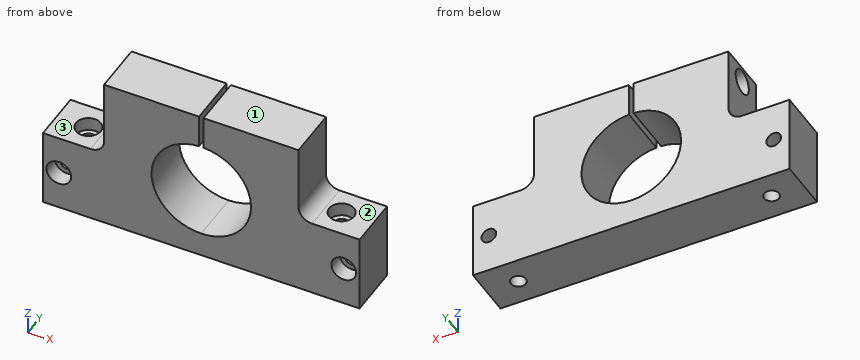
from build123d import *

# Parameters (mm, degrees)
DODANIE_WYCI_GNI_CIE1_DEPTH                        = 23
ZAOKR_GLENIE1_R                                    = 6
POG_BIENIE_START                                   = 27
POG_BIENIE_WALCOWE_POD_M6_WKR_T_DO_C_2_R           = 3.25
POG_BIENIE_WALCOWE_POD_M6_WKR_T_DO_CZ_CI_DEPTH     = 42
POG_BIENIE_WALCOWE_POD_M6_WKR_T_DO_C_3_O_R         = 5.5
POG_BIENIE_WALCOWE_POD_M6_WKR_T_DO_C_3_O_R_2       = 3.25
POG_BIENIE_WALCOWE_POD_M6_WKR_T_DO_C_3_DEPTH       = 7
OTW_R_GWINTOWANY_M6X1_01_D                         = 5
OTW_R_GWINTOWANY_M6X1_01_DEPTH                     = 17
OTW_R_GWINTOWANY_M6X1_01_TIP                       = 1.502151548
POG_BIENIE_WALCOWE_POD_M6_WKR_T_DO_C_4_D           = 6.6
POG_BIENIE_WALCOWE_POD_M6_WKR_T_DO_C_4_CBORE_D     = 11
POG_BIENIE_WALCOWE_POD_M6_WKR_T_DO_C_4_CBORE_DEPTH = 6
POG_BIENIE_WALCOWE_POD_M6_WKR_T_DO_C_5_D           = 6.5
POG_BIENIE_WALCOWE_POD_M6_WKR_T_DO_C_5_CBORE_D     = 11
POG_BIENIE_WALCOWE_POD_M6_WKR_T_DO_C_5_CBORE_DEPTH = 7


# Read off the part's stored shape, not the designer's step: Pogłębienie walcowe pod M6 Wkręt do części metalowych z łbem sześciokątnym1
with BuildPart() as part:
    # Szkic1 → Dodanie-wyciągnięcie1 (new body)
    with BuildSketch(Plane(origin=(0, 0, 0), x_dir=(1, 0, 0), z_dir=(0, 1, 0))):
        with BuildLine():
            Line((0, 0), (0, -35))
            Line((0, -35), (27, -35))
            Line((27, -35), (27, -70))
            Line((27, -70), (69, -70))
            Line((69, -70), (69, -54.977260976))
            ThreePointArc((69, -54.977260976), (48.005685491, -32.499870751), (70, -11))
            Line((70, -11), (70, 0))
            Line((70, 0), (0, 0))
        make_face()
        with BuildLine():
            Line((140, 0), (70, 0))
            Line((70, 0), (70, -11))
            ThreePointArc((70, -11), (91.994314509, -32.499870751), (71, -54.977260976))
            Line((71, -54.977260976), (71, -70))
            Line((71, -70), (113, -70))
            Line((113, -70), (113, -35))
            Line((113, -35), (140, -35))
            Line((140, -35), (140, 0))
        make_face()
    extrude(amount=DODANIE_WYCI_GNI_CIE1_DEPTH)

    # Zaokrąglenie1
    zaokr_glenie1_edges = [part.edges().sort_by_distance(p)[0] for p in [
        (27, 11.5, 35),
        (113, 11.5, 35),
    ]]
    fillet(zaokr_glenie1_edges, radius=ZAOKR_GLENIE1_R)

    # Pog_bienie walcowe pod M6 Wkr_t do c 2 → Pog_bienie walcowe pod M6 Wkr_t do cz_ci (cut)
    with BuildSketch(Plane.YZ.offset(POG_BIENIE_START)):
        with Locations((11.5, 63)):
            Circle(POG_BIENIE_WALCOWE_POD_M6_WKR_T_DO_C_2_R)
    extrude(amount=POG_BIENIE_WALCOWE_POD_M6_WKR_T_DO_CZ_CI_DEPTH, mode=Mode.SUBTRACT)

    # Pog_bienie walcowe pod M6 Wkr_t do c 3 o → Pog_bienie walcowe pod M6 Wkr_t do c 3 (cut)
    with BuildSketch(Plane.YZ.offset(POG_BIENIE_START)):
        with Locations((11.5, 63)):
            Circle(POG_BIENIE_WALCOWE_POD_M6_WKR_T_DO_C_3_O_R)
        with Locations((11.5, 63)):
            Circle(POG_BIENIE_WALCOWE_POD_M6_WKR_T_DO_C_3_O_R_2, mode=Mode.SUBTRACT)
    extrude(amount=POG_BIENIE_WALCOWE_POD_M6_WKR_T_DO_C_3_DEPTH, mode=Mode.SUBTRACT)

    # Otwór gwintowany M6x1.01
    with Locations(Plane.ZY.offset(-71)):
        with Locations((63, 11.5)):
            Hole(OTW_R_GWINTOWANY_M6X1_01_D / 2, depth=OTW_R_GWINTOWANY_M6X1_01_DEPTH)
            with Locations((0, 0, -(OTW_R_GWINTOWANY_M6X1_01_DEPTH + OTW_R_GWINTOWANY_M6X1_01_TIP / 2))):  # 118° drill point
                Cone(0, OTW_R_GWINTOWANY_M6X1_01_D / 2, OTW_R_GWINTOWANY_M6X1_01_TIP, mode=Mode.SUBTRACT)

    # Pog_bienie walcowe pod M6 Wkr_t do c 4 (through all)
    with Locations(Plane.XY.offset(35)):
        with Locations((14, 11.5), (126, 11.5)):
            CounterBoreHole(POG_BIENIE_WALCOWE_POD_M6_WKR_T_DO_C_4_D / 2, POG_BIENIE_WALCOWE_POD_M6_WKR_T_DO_C_4_CBORE_D / 2, POG_BIENIE_WALCOWE_POD_M6_WKR_T_DO_C_4_CBORE_DEPTH)

    # Pog_bienie walcowe pod M6 Wkr_t do c 5 (through all)
    with Locations(Plane(origin=(0, 0, 0), x_dir=(-1, 0, 0), z_dir=(0, -1, 0))):
        with Locations((-7, -17.5), (-133, -17.5)):
            CounterBoreHole(POG_BIENIE_WALCOWE_POD_M6_WKR_T_DO_C_5_D / 2, POG_BIENIE_WALCOWE_POD_M6_WKR_T_DO_C_5_CBORE_D / 2, POG_BIENIE_WALCOWE_POD_M6_WKR_T_DO_C_5_CBORE_DEPTH)


solid = part.part
The listing builds one solid part. Answer for the finished solid, in the listing's coordinates (mm). Face numbers are marked on the shaded views. A direction names the side the tool comes from. Coordinates: 2 decimals unless noted, no trailing zeros. Loops run counter-clockwise (first coordinate to the right, second up) from the corner with the lowest first, then second, coordinate; pieces in that order, holes last. Notation, with made-up numbers: M -28,-35.75 L 1,-35.75 A9 cw 1,-19.75 Z; hole C 51,76.25 d8. An arc over 180 degrees is marked long. Answer in a Markdown table with one row per item.
1) Find the intervals of material crossed by probe 1 along Z at (x, y) = (133, 17); probe 2 along X at (y, z) = (3.25, 17.5); probe 3 along Y at (x, z) = (126, 18.5), in increasing order.
Answers below:
| item | result |
|---|---|
| probe 1 | 0 to 14.25, 20.75 to 35 |
| probe 2 | 0 to 1.5, 12.5 to 54.39, 85.61 to 127.5, 138.5 to 140 |
| probe 3 | 0 to 8.2, 14.8 to 23 |
2) Find section A-A (z = 33). Determine the outline of the cut face in (x, y), then the cut area to 3 significant figures.
Answers below:
| item | result |
|---|---|
| outline | M 0,0 L 48,0 L 48,23 L 0,23 Z; M 92,0 L 140,0 L 140,23 L 92,23 Z; hole C 14,11.5 d11; hole C 126,11.5 d11 |
| area | 2,020 mm^2 |
3) Which of the six approach directions +Z, -Z, +X, -X, +Y, -Y give full straight-line access (tool end or side, diameter ignored) to the marked faces 1, 2 and 3?
Answers below:
| item | result |
|---|---|
| face 1 | +Z, +X, -X, +Y, -Y |
| face 2 | +Z, +X, +Y, -Y |
| face 3 | +Z, -X, +Y, -Y |
4) Find section C-C (z = 17.5). Determine the outline of the cut face in (x, y).
Answers below:
| item | result |
|---|---|
| outline | M 0,0 L 1.5,0 L 1.5,7 L 3.75,7 L 3.75,23 L 0,23 Z; M 10.25,7 L 12.5,7 L 12.5,0 L 54.39,0 L 54.39,23 L 10.25,23 Z; M 85.61,0 L 127.5,0 L 127.5,7 L 129.75,7 L 129.75,23 L 85.61,23 Z; M 136.25,7 L 138.5,7 L 138.5,0 L 140,0 L 140,23 L 136.25,23 Z; hole C 14,11.5 d6.6; hole C 126,11.5 d6.6 |
5) Find section D-D (y = 2.25). Determine the outline of the cut face in (x, z), then the cut area to 3 significant figures.
Answers below:
| item | result |
|---|---|
| outline | M 0,0 L 140,0 L 140,35 L 119,35 A6 cw 113,41 L 113,70 L 71,70 L 71,54.98 A22 cw long 69,54.98 L 69,70 L 27,70 L 27,41 A6 cw 21,35 L 0,35 Z; hole C 7,17.5 d11; hole C 133,17.5 d11 |
| area | 6,180 mm^2 |
6) Given pin 1 (6 mm diameter, centred on y = 5.5, z = 52, fed in from -X); pin 2 (6.5 mm diameter, centred on x = 130.5, y = 8.5, fed in from +Z); pin 3 (4.5 mm diameter, centred on y = 9, z = 64.5, fed in from -X), each flat-ended and moving along its own axis, determine where each tip first touches the part or whether it passes through.
Answers below:
| item | result |
|---|---|
| pin 1 | x = 27 |
| pin 2 | z = 35 |
| pin 3 | x = 34 |
7) Find section B-B (x = 126). Determine the outline of the cut face in (y, z).
Answers below:
| item | result |
|---|---|
| outline | M 0,0 L 8.2,0 L 8.2,29 L 6,29 L 6,35 L 0,35 Z; M 14.8,0 L 23,0 L 23,35 L 17,35 L 17,29 L 14.8,29 Z |
